```python
from build123d import *

# Parameters (mm, degrees)
F0_R     = 2.25
F1_DEPTH = 2
F2_DEPTH = 5
F3_DEPTH = 3
F4_SIZE  = 0.99999


# Not quite as in the source:
# - a fillet or chamfer is up to 0.001 mm smaller than in the source, because OpenCascade refuses the exact size


with BuildPart() as f1:
    # F0 (on Top) → F1 (new body)
    with BuildSketch(Plane.XY):
        with BuildLine():
            ThreePointArc((4, -13.416407865), (11.2249721603, -8.3666002653), (14, 0))
            ThreePointArc((14, 0), (-8.3666002653, 11.2249721603), (-4, -13.416407865))
            Line((-4, -13.416407865), (-4, -11.5785361769))
            ThreePointArc((-4, -11.5785361769), (-7.1085336041, 9.9765349696), (12.25, 0))
            ThreePointArc((12.25, 0), (9.9765349696, -7.1085336041), (4, -11.5785361769))
            Line((4, -11.5785361769), (4, -13.416407865))
        make_face()
        with BuildLine():
            ThreePointArc((12.25, 0), (-7.1085336041, 9.9765349696), (-4, -11.5785361769))
            Line((-4, -11.5785361769), (-4, -7))
            Line((-4, -7), (4, -7))
            Line((4, -7), (4, -11.5785361769))
            ThreePointArc((4, -11.5785361769), (9.9765349696, -7.1085336041), (12.25, 0))
        make_face()
        Circle(F0_R, mode=Mode.SUBTRACT)
        Circle(F0_R)
    extrude(amount=F1_DEPTH)

    # F0 (on Top) → F2 (join)
    with BuildSketch(Plane.XY):
        with BuildLine():
            ThreePointArc((4, -13.416407865), (11.2249721603, -8.3666002653), (14, 0))
            ThreePointArc((14, 0), (-8.3666002653, 11.2249721603), (-4, -13.416407865))
            Line((-4, -13.416407865), (-4, -11.5785361769))
            ThreePointArc((-4, -11.5785361769), (-7.1085336041, 9.9765349696), (12.25, 0))
            ThreePointArc((12.25, 0), (9.9765349696, -7.1085336041), (4, -11.5785361769))
            Line((4, -11.5785361769), (4, -13.416407865))
        make_face()
    extrude(amount=F2_DEPTH)

    # F0 (on Top) → F3 (join)
    with BuildSketch(Plane.XY):
        Circle(F0_R)
    extrude(amount=F3_DEPTH)

    # F4 (size 1 in the source; OpenCascade refuses exactly that, so slightly less here)
    f4_edges = [f1.edges().sort_by_distance(p)[0] for p in [
        (0, 14, 0),
        (-7.108534, 9.976535, 5),
        (0, -7, 2),
        (-4, -9.289268, 2),
        (4, -9.289268, 2),
    ]]
    chamfer(f4_edges, length=F4_SIZE)


solid = f1.part
```
CAD build for the part. Positions are in the model's coordinates, mm. A direction names the side the tool comes from. Round coordinates to 2 decimals unless told otherwise and drop trailing zeros. Order: outer loops, then holes, each group sorted by start corner. A loop starts at its lowest first (then second) coordinate and runs counter-clockwise, first axis right, second up.
Q1. Slice it at B-B (z = 2.6). Write the cut outline in (x, y).
Q2. Drop flat-ended pins along their axis: pin 1 (2.5 mm diameter, centred on y = -11.5, z = 1.5, fed in from -X); pin 2 (2.5 mm diameter, centred on y = -10.5, z = 3, fed in from +X); pin 3 (1.3 mm diameter, centred on x = -0.5, y = -1, fed in from +Z); pin 4 (4 mm diameter, centred on x = 7.5, y = -2, fed in from -Z). Give the stop position or say it passes through.
Q3. Slice it at A-A (x = 0). Write the cut outline in (y, z), and give its area (4 significant figures).
Q4. Two-plate mould, pull along X, no slides. Class faces 1 (the cylindrical face through (-0.29, 2.23, 2.49)), 2 (the flat face through (-8, 11, 5)), 3 (the conical face through (0.53, 13.16, 0.17)): pulls with the +X half, pulls with the -X half, needs draft (parallel to the pull), parting line crosses it, or undercut.
Q5. Which spindle directions (+Z, -Z, +X, -X, +Y, -Y) get a long thin tool onto all of the face, cutting with end or side? Do faces 4 (the flat face through (-0.1, -7, 0.5)), 5 (the cylindrical face through (0.56, 13.99, 2.97)), 6 (the flat face through (0, 0, 3)), 7 (the flat face through (0, 0, 0)), 8 (the flat face through (4.5, -8.8, 1.5)). Say none if no direction does.
Q6. Wall check: L1, parallel to Y at x = 0, z = 2.3; L2, parallel to Z at x = 12, y = -2; L3, parallel to Y at x = 0, z = 3.1. Give the ranges that are in metal, low to high.
Q7. Slice it at C-C (z = 0.55). Write the cut outline in (x, y).
Results below:
1. outline: (-4, -13.42) - (-4, -11.58) arc R12.25 cw (long way) to (4, -11.58) - (4, -13.42) arc R14 ccw (long way) to start; circle Ø4.5 at (0, 0)
2. pin 1: stops at x = -9.54
2. pin 2: stops at x = 10.51
2. pin 3: stops at z = 3
2. pin 4: stops at z = 0
3. outline: (-7, 0) - (13, 0) - (14, 1) - (14, 5) - (13.25, 5) - (12.25, 4) - (12.25, 2) - (2.25, 2) - (2.25, 3) - (-2.25, 3) - (-2.25, 2) - (-6, 2) - (-7, 1) - close
3. area: 50.25 mm2
4. face 1: undercut
4. face 2: needs draft
4. face 3: parting line crosses it
5. face 4: +Z, -Z, -Y
5. face 5: +Z, -Z
5. face 6: +Z, -Y
5. face 7: -Z, +X, -X, +Y, -Y
5. face 8: +Z
6. L1: y = -2.25 to 2.25, 12.25 to 14
6. L2: z = 0 to 2
6. L3: y = 12.25 to 14
7. outline: (-4, -12.95) - (-4, -7) - (4, -7) - (4, -12.95) arc R13.55 ccw (long way) to start
